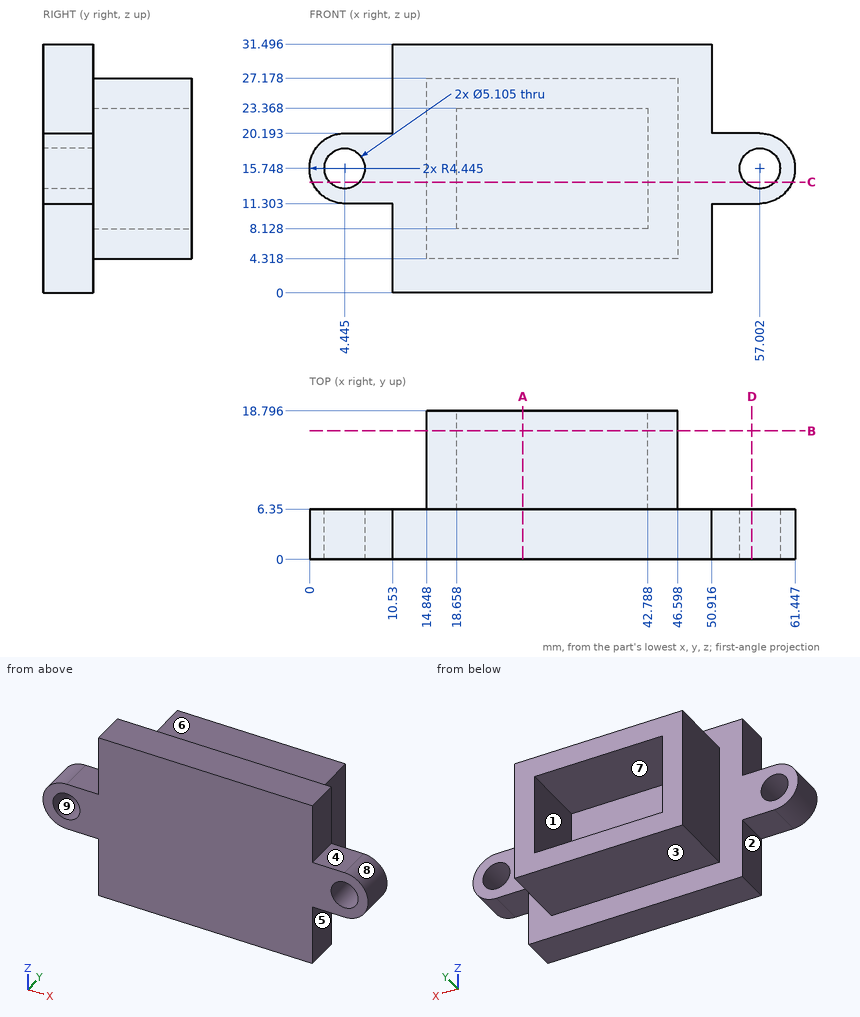
Can you work these out from the drawing? Everything is in mm from the part's minimum corner. A direction names the side the tool comes from. Round coordinates to 2 decimals unless told otherwise and drop trailing zeros. Loops run counter-clockwise (first coordinate to the right, second up) from the corner with the lowest first, then second, coordinate; pieces in that order, holes last. Notation, with made-up numbers: M -9.75,21.25 L 32.25,21.25 A14 ccw 32.25,32.25 Z; hole C -12.75,1 d5. An arc over 180 degrees is marked long. Answer in a Markdown table with one row per item.
1. If we section it at D-D, the plane x = 56: Please give me the cut outline in (y, z).
Established:
| item | result |
|---|---|
| outline | M 0,11.3 L 6.35,11.3 L 6.35,13.4 L 0,13.4 Z; M 0,18.1 L 6.35,18.1 L 6.35,20.19 L 0,20.19 Z |
2. If we section it at B-B, the plane y = 16.25: Please give me the cut outline in (x, z).
Established:
| item | result |
|---|---|
| outline | M 14.85,4.32 L 46.6,4.32 L 46.6,27.18 L 14.85,27.18 Z; hole M 18.66,8.13 L 42.79,8.13 L 42.79,23.37 L 18.66,23.37 Z |
3. If we section it at A-A, the plane x = 27: Please give me the cut outline in (y, z).
Established:
| item | result |
|---|---|
| outline | M 0,0 L 6.35,0 L 6.35,4.32 L 18.8,4.32 L 18.8,8.13 L 6.35,8.13 L 6.35,23.37 L 18.8,23.37 L 18.8,27.18 L 6.35,27.18 L 6.35,31.5 L 0,31.5 Z |
4. On a 3-axis mill with a long thin cutter (end or side, diameter ignored), from which of +Z, -Z, +X, -X, +Y, -Y can I reach the whole of each face in a straight line? I mean the marked faces 1, 2, 3, 4 and 5. Say none if no direction works.
Established:
| item | result |
|---|---|
| face 1 | +Y |
| face 2 | -Z, -X, +Y, -Y |
| face 3 | -Z, +X, -X, +Y |
| face 4 | +Z, +X, +Y, -Y |
| face 5 | -Z, +X, +Y, -Y |
5. If we section it at C-C, the plane z = 14: Give the number of separate pieces and of enclosed holes in the cut face, plus the area to 3 significant figures.
Established:
| item | result |
|---|---|
| separate pieces | 3 |
| enclosed holes | 0 |
| area | 433 mm² |
6. Please list where these lines run through material, in increasing order: line 1 (Z direction, x = 25.5, y = 13); line 2 (Z direction, x = 4.5, y = 1.25); line 3 (X direction, y = 17.75, z = 15). Write a range as from..to.
Established:
| item | result |
|---|---|
| line 1 | 4.32..8.13, 23.37..27.18 |
| line 2 | 11.3..13.2, 18.3..20.19 |
| line 3 | 14.85..18.66, 42.79..46.6 |
7. Thinking about a two-plate mould opening in Z: for the marked faces 6, 7, 8 and 9, which applies, pulls with the +Z half, pulls with the -Z half, needs draft (parallel to the pull), parting line crosses it, or undercut?
Established:
| item | result |
|---|---|
| face 6 | pulls with the +Z half |
| face 7 | undercut |
| face 8 | parting line crosses it |
| face 9 | undercut |
8. I'm going to push flat-ended pins straight in: pin 1 Ø3.5 at (y, z) = (12, 18.5) entering from +X; pin 2 Ø6 at (x, y) = (27, 14.5) entering from +Z; pin 3 Ø3 at (x, y) = (35.5, 14) entering from -Z. Where does each tip first touch, or does it pass through?
Established:
| item | result |
|---|---|
| pin 1 | x = 46.6 |
| pin 2 | z = 27.18 |
| pin 3 | z = 4.32 |
